Can you work these out from the model? Positions are in its coordinate system, mm. A direction names the side the tool comes from. Give positions to 0.01 mm unless a question says otherwise; leave off trailing zeros. Loops run counter-clockwise (first coordinate to the right, second up) from the corner with the lowest first, then second, coordinate; pieces in that order, holes last.
from build123d import *

# Parameters (mm, degrees)
F1_DEPTH = 7
F2_DEPTH = 10
F3_R     = 7


with BuildPart() as f1:
    # F0 (on Top) → F1 (new body, symmetric)
    with BuildSketch(Plane.XY):
        with BuildLine():
            ThreePointArc((-11.358531, 3.689624), (-27.896694, 20.489591), (-34.898927, 43))
            Line((-34.898927, 43), (-206.909318, -110.62962))
            ThreePointArc((-206.909318, -110.62962), (-208.702535, -142.398857), (-176.933299, -144.192073))
            Line((-176.933299, -144.192073), (-11.358531, 3.689624))
        make_face()
    extrude(amount=F1_DEPTH, both=True)

    # F0 (on Top) → F2 (join, symmetric)
    with BuildSketch(Plane.XY):
        with BuildLine():
            Line((5, 62), (35, 62))
            ThreePointArc((35, 62), (21.704163, 80.131071), (0, 86))
            ThreePointArc((0, 86), (-5.902823, 84.843409), (-11.358531, 82.310376))
            ThreePointArc((-11.358531, 82.310376), (-27.896694, 65.510409), (-34.898927, 43))
            ThreePointArc((-34.898927, 43), (-27.896694, 20.489591), (-11.358531, 3.689624))
            ThreePointArc((-11.358531, 3.689624), (-5.902823, 1.156591), (0, 0))
            ThreePointArc((0, 0), (21.704163, 5.868929), (35, 24))
            Line((35, 24), (5, 24))
            ThreePointArc((5, 24), (-5.909463, 43), (5, 62))
        make_face()
    extrude(amount=F2_DEPTH, both=True)

    # F3
    f3_edges = [f1.edges().sort_by_distance(p)[0] for p in [
        (-34.898927, 43, 0),
        (-11.358531, 3.689624, 0),
    ]]
    fillet(f3_edges, radius=F3_R)


solid = f1.part
(1) Will these pins go through, and if not, where does the flat tip stop? P1, Ø6, axis at x = -75, y = 6, coming from the +Z side; P2, Ø2, axis at y = -89, z = 5, coming from the +X side; P3, Ø1.5, axis at y = -53.5, z = -5.5, coming from the +X side.
Returned:
P1: stops at z = 7
P2: stops at x = -114.02
P3: stops at x = -74.55
(2) Please list where these lines run through material, in increasing order: probe 1 along Z at (x, y) = (-53.5, 3); probe 2 along Y at (x, z) = (-1.5, -0.5); probe 3 along Y at (x, z) = (-81.5, -6.75).
Returned:
probe 1: z = -7 to 7
probe 2: y = 0.16 to 29.79, 56.21 to 85.84
probe 3: y = -58.96 to 1.38
(3) Which directions (+Z, -Z, +X, -X, +Y, -Y) give clear straight access to the entire face, cutting with the end or side of a thin tool? Please do faces 5 (the flat face through (-8, 44, -10)), 6 (the flat face through (20, 62, 0)), 7 (the cylindrical face through (-28.07, 20.78, 8.52)).
Returned:
face 5: -Z, +X, -X, +Y, -Y
face 6: +Z, -Z, +X
face 7: +Z, -X, -Y
(4) Suppose I cut it at A-A on x = -30. List the corners of the cut face in (y, z) for me.
Returned:
outline: (-12.96, -7) - (24.38, -7) - (24.38, -10) - (61.62, -10) - (61.62, 10) - (24.38, 10) - (24.38, 7) - (-12.96, 7) - close
(5) Suppose I cut it at D-D on x = -136. List the corners of the cut face in (y, z) for me, plus the area to 3 significant figures.
Returned:
outline: (-107.63, -7) - (-47.3, -7) - (-47.3, 7) - (-107.63, 7) - close
area: 845 mm2
(6) Thinking about a two-plate mould opening in Y: for faces 1 (the cylindrical face through (-28.07, 20.78, -8.48)), 2 (the flat face through (20, 24, 0)), 3 (the cylindrical face through (-5.907, 42.679, 0.14)), 4 (the flat face through (-8, 44, 10)), which applies, pulls with the +Y half, pulls with the -Y half, needs draft (parallel to the pull), parting line crosses it, or undercut?
Returned:
face 1: pulls with the -Y half
face 2: undercut
face 3: undercut
face 4: needs draft
(7) Suppose I cut it at C-C on y = -29. List the corners of the cut face in (x, z) for me, plus the area to 3 significant figures.
Returned:
outline: (-115.51, -7) - (-47.96, -7) - (-47.96, 7) - (-115.51, 7) - close
area: 946 mm2
(8) Suppose I cut it at B-B on z = 1. List the corners of the cut face in (x, y) for me.
Returned:
outline: (-206.91, -110.63) arc R22.5 ccw to (-176.93, -144.19) - (-14.91, 0.52) arc R7 cw to (-7.61, 1.78) arc R25 ccw to (0, 0) arc R34 ccw to (35, 24) - (5, 24) arc R22 cw to (5, 62) - (35, 62) arc R34 ccw to (0, 86) arc R25 ccw to (-11.36, 82.31) arc R50 ccw to (-34.67, 45.58) arc R7 cw to (-36.96, 41.16) - close
